Check sheet for the drawn part. Datum: minimum x, y, z corner. Units: mm. Coordinates: 2 decimals unless noted, no trailing zeros. Order: outer loops, then holes, each group sorted by start corner. A loop starts at its lowest first (then second) coordinate and runs counter-clockwise, first axis right, second up. Notation, with made-up numbers: M -29,10.5 L 6,10.5 A30 ccw 6,44.5 Z; hole C -29,-34 d4. An arc over 180 degrees is marked long. Return JSON: item names as keys, results as strings. Group by question number.
Q1. Section check D-D, the plane y = 78. Enter the section's corners in (x, z), then the cut area to 3 significant figures.
Q2. Go/stop test with a flat-tipped pin: pin 1 Ø3.5 at (x, y) = (42.5, 14) entering from -Z. Record where the tip stops, or that it passes through.
Q3. Section check A-A, the plane x = 41.5. Enter the section's corners in (y, z) (3 decimals), then the cut area to 3 significant figures.
Q4. Section check C-C, the plane z = 3.5. Enter the section's corners in (x, y) (3 decimals).
Q5. Section check B-B, the plane y = 16.5. Enter the section's corners in (x, z) (3 decimals).
Q6. Thickness scan on probe 1 along Y at (x, z) = (5, 3.5); probe 2 along Y at (x, z) = (41.5, 7.3); probe 3 along X at (y, z) = (66.5, 2.3) (3 decimals). Record the ranges inside material, lowest first.
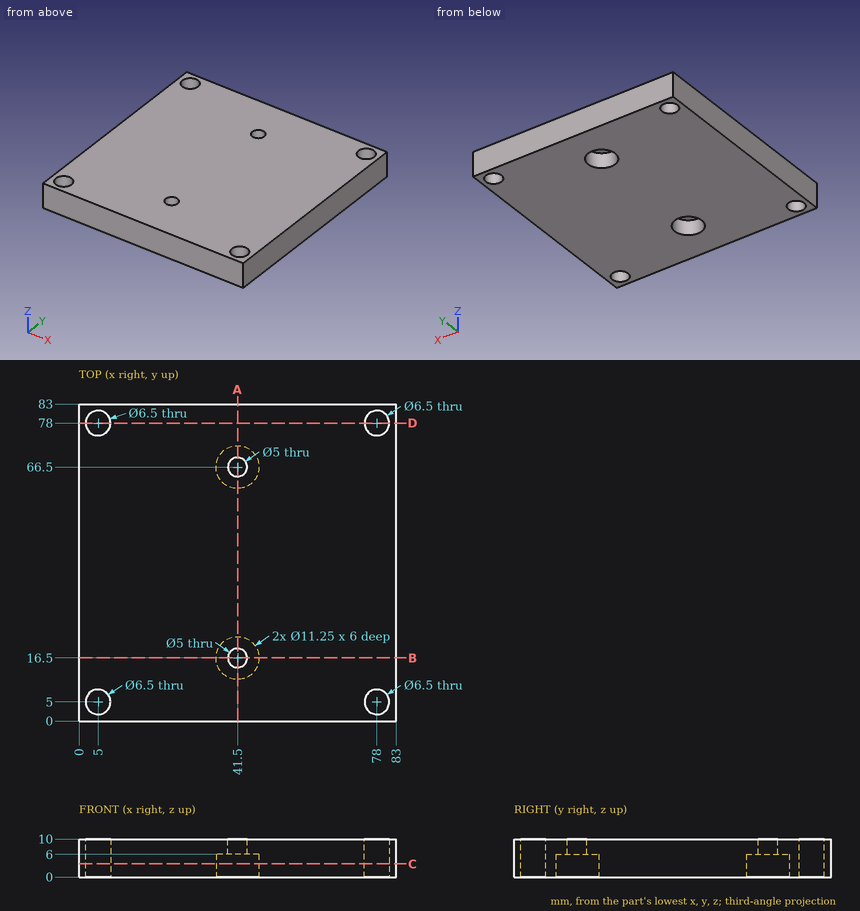
Numbers:
{
 "1": {"outline": "M 0,0 L 1.75,0 L 1.75,10 L 0,10 Z; M 8.25,0 L 74.75,0 L 74.75,10 L 8.25,10 Z; M 81.25,0 L 83,0 L 83,10 L 81.25,10 Z", "area": "700 mm2"},
 "2": {"pin 1": "stops at z = 6"},
 "3": {"outline": "M 0,0 L 10.875,0 L 10.875,6 L 14,6 L 14,10 L 0,10 Z; M 19,6 L 22.125,6 L 22.125,0 L 60.875,0 L 60.875,6 L 64,6 L 64,10 L 19,10 Z; M 69,6 L 72.125,6 L 72.125,0 L 83,0 L 83,10 L 69,10 Z", "area": "655 mm2"},
 "4": {"outline": "M 0,0 L 83,0 L 83,83 L 0,83 Z; hole C 5,5 d6.5; hole C 5,78 d6.5; hole C 41.5,16.5 d11.25; hole C 41.5,66.5 d11.25; hole C 78,5 d6.5; hole C 78,78 d6.5"},
 "5": {"outline": "M 0,0 L 35.875,0 L 35.875,6 L 39,6 L 39,10 L 0,10 Z; M 44,6 L 47.125,6 L 47.125,0 L 83,0 L 83,10 L 44,10 Z"},
 "6": {"probe 1": "y = 0 to 1.75, 8.25 to 74.75, 81.25 to 83", "probe 2": "y = 0 to 14, 19 to 64, 69 to 83", "probe 3": "x = 0 to 35.875, 47.125 to 83"}
}
